Build history of the part. All positions in model axes, mm. A direction names the side the tool comes from. Give positions to 0.01 mm unless a question says otherwise; leave off trailing zeros. Write each loop counter-clockwise with the first axis right and the second up, starting at its lowest first coordinate (ties: lowest second). Pieces come first, ordered by that corner, then holes.
Autodesk Inventor part; units mm, degrees
ref_plane "YZ Plane" through (0, 0, 0) normal (1, 0, 0) x (0, 1, 0)
ref_plane "XZ Plane" through (0, 0, 0) normal (0, 1, 0) x (-1, 0, 0)
ref_plane "XY Plane" through (0, 0, 0) normal (0, 0, 1) x (1, 0, 0)
sketch "Sketch1" plane through (0, 0, 0) normal (0, 1, 0) x (-1, 0, 0)
  line L0 (-52.5, -52.5) -> (52.5, -52.5)
  line L1 (52.5, -52.5) -> (52.5, 52.5)
  line L2 (52.5, 52.5) -> (-52.5, 52.5)
  line L3 (-52.5, 52.5) -> (-52.5, -52.5)
  line L4 (-52.5, -52.5) -> (52.5, 52.5) construction
  line L5 (52.5, -52.5) -> (-52.5, 52.5) construction
  point P0 (0, 0)
extrude "Extrusion1" add sketch "Sketch1" along normal blind 5
sketch "Sketch4" plane through (0, 5, 0) normal (0, 1, 0) x (1, 0, 0)
  line L0 (-52.5, 52.5) -> (-52.5, -52.5)
  line L1 (52.5, 52.5) -> (-52.5, 52.5)
  line L2 (-52.5, 52.5) -> (-52.5, -52.5)
  line L3 (-52.5, -52.5) -> (52.5, -52.5)
  line L4 (52.5, -52.5) -> (52.5, 52.5)
  line L5 (52.5, 52.5) -> (-52.5, -52.5) construction
  line L6 (-52.5, 52.5) -> (52.5, -52.5) construction
  line L7 (50, 50) -> (-50, 50)
  line L8 (-50, 50) -> (-50, -50)
  line L9 (-50, -50) -> (50, -50)
  line L10 (50, -50) -> (50, 50)
  line L11 (50, 50) -> (-50, -50) construction
  line L12 (-50, 50) -> (50, -50) construction
  line L13 (52.5, 52.5) -> (-52.5, 52.5)
  line L14 (-52.5, 52.5) -> (-52.5, -52.5)
  line L15 (-52.5, -52.5) -> (52.5, -52.5)
  line L16 (52.5, -52.5) -> (52.5, 52.5)
  line L17 (52.5, 52.5) -> (-52.5, -52.5) construction
  line L18 (-52.5, 52.5) -> (52.5, -52.5) construction
  point P0 (0, 0)
extrude "Extrusion2" add sketch "Sketch4" along normal blind 40
fillet "Fillet1" radius 2.5 4 edges at (0, 45, -50) (-50, 45, 0) (0, 45, 50) (50, 45, 0)
sketch "Sketch5" plane through (0, 5, 0) normal (0, 1, 0) x (1, 0, 0)
  circle A0 centre (0, 0) radius 2.5
  dimension "d12" = 5
extrude "Extrusion3" cut sketch "Sketch5" against normal blind 10
sketch "Sketch6" plane through (0, 5, 0) normal (0, 1, 0) x (1, 0, 0)
  circle A0 centre (0, 0) radius 4.25
  dimension "d15" = 8.5
extrude "Extrusion4" cut sketch "Sketch6" against normal blind 2
properties part number "KwadratP"
(1) Mould opens along X. For faces 3 (the face through (-1, 22, 52.5)), 4 (the face through (-50, 23, -1)), 5 (the face through (-52.5, 22, -1)) say: +X half, -X half, draft (parallel to the pull), parting line (faces both ways), or undercut.
(2) 3-axis set-ups, long thin cutter, end or side, ignore diameter. For faces 1 (the face through (52.5, 22, 1)), 2 (the face through (1, 5, 12)): which of +Z, -Z, +X, -X, +Y, -Y reach the whole face in a straight line?
(3) Drop a flat-ended pin along its axis: pin 1 (7 mm diameter, centred on x = 0, z = -1, fed in from +Y). Give the stop position or say it passes through.
(4) Probe line 1 (X direction, y = 31.5, z = 28); line 2 (Z direction, x = 0, y = 4.4). List the from-to ranges inside material, lowest first.
(5) Saw through at C-C, the plane y = 21. List the corners of the cut face in (x, z).
Computed values:
1. face 3: draft
1. face 4: undercut
1. face 5: -X half
2. face 1: +Z, -Z, +X, +Y, -Y
2. face 2: +Y
3. pin 1: stops at y = 5
4. line 1: x = -52.5 to -50, 50 to 52.5
4. line 2: z = -52.5 to -4.25, 4.25 to 52.5
5. outline: (-52.5, -52.5) - (52.5, -52.5) - (52.5, 52.5) - (-52.5, 52.5) - close; hole (-50, -50) - (50, -50) - (50, 50) - (-50, 50) - close
